Input: part model. Units: mm. Frame: model coordinates. Face numbers are marked on the shaded views. Coordinates: 2 decimals unless noted, no trailing zeros. Write each loop counter-clockwise with the first axis right and the second up, starting at its lowest first coordinate (ties: lowest second). Pieces come first, ordered by that corner, then holes. Notation, with made-up numbers: (72.25, -17.75) - (121.25, -17.75) arc R32 cw to (121.25, 19.25) - close; hole circle Ø4 at (89, 32). An arc over 180 degrees is marked (long way). Put each result on its own line as item: value. Start each with the question number.
1. Cut plane B-B, the plane z = 54.5. Return loops of the section in (x, y).
2. Cut plane C-C, the plane z = -13.5. Return loops of the section in (x, y), and give its area (3 significant figures).
3. Cut plane A-A, the plane y = 0. Return loops of the section in (x, z), and give its area (3 significant figures).
4. Line query: line 1 (Y direction, x = 7.75, z = 0); line 2 (Z direction, x = 14.5, y = -32); line 3 (Z direction, x = 14.25, y = 24.5). Output: solid intervals per line, ascending.
5. Cut plane D-D, the plane x = 11.75. Count the separate pieces of the cut face and the enclosed holes in it, and give its area (3 significant figures).
6. Pull-direction query (Z, two-part tool) for the marked faces 1, 2 and 3; classes: released by +Z, released by -Z, zero draft, split by the parting line, or undercut.
7. Pin query (flat end, axial travel): pin 1 (10 mm diameter, centred on x = 15.5, z = 31, fed in from +Y); pin 2 (3.5 mm diameter, centred on x = 10.5, y = 33.5, fed in from -Z); pin 3 (4 mm diameter, centred on x = 14, z = 30, fed in from +Y). Return the tip coordinate at first contact, or that it passes through.
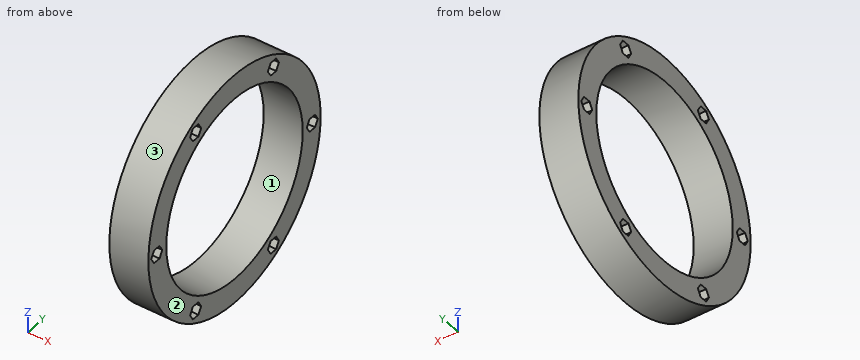
from build123d import *

# Parameters (mm, degrees)
SKETCH1_R           = 72
SKETCH1_R_2         = 57
BOSS_EXTRUDE1_DEPTH = 24
CUT_EXTRUDE1_DEPTH  = 24


with BuildPart() as part:
    # Sketch1 → Boss-Extrude1 (new body)
    with BuildSketch(Plane(origin=(0, 0, 0), x_dir=(0, 0, -1), z_dir=(1, 0, 0))):
        Circle(SKETCH1_R)
        Circle(SKETCH1_R_2, mode=Mode.SUBTRACT)
    extrude(amount=BOSS_EXTRUDE1_DEPTH)

    # Sketch2 → Cut-Extrude1 (cut)
    with BuildSketch(Plane(origin=(24, 0, 0), x_dir=(0, 0, -1), z_dir=(1, 0, 0))):
        Polygon((52.291651246, 30.190598923), (56.291651246, 27.881197846), (60.291651246, 30.190598923), (60.291651246, 34.809401077), (56.291651246, 37.118802154), (52.291651246, 34.809401077), align=None)
        Polygon((0, 60.381197846), (4, 62.690598923), (4, 67.309401077), (0, 69.618802154), (-4, 67.309401077), (-4, 62.690598923), align=None)
        Polygon((52.291651246, -30.190598923), (52.291651246, -34.809401077), (56.291651246, -37.118802154), (60.291651246, -34.809401077), (60.291651246, -30.190598923), (56.291651246, -27.881197846), align=None)
        Polygon((0, -60.381197846), (-4, -62.690598923), (-4, -67.309401077), (0, -69.618802154), (4, -67.309401077), (4, -62.690598923), align=None)
        Polygon((-52.291651246, -30.190598923), (-56.291651246, -27.881197846), (-60.291651246, -30.190598923), (-60.291651246, -34.809401077), (-56.291651246, -37.118802154), (-52.291651246, -34.809401077), align=None)
        Polygon((-52.291651246, 30.190598923), (-52.291651246, 34.809401077), (-56.291651246, 37.118802154), (-60.291651246, 34.809401077), (-60.291651246, 30.190598923), (-56.291651246, 27.881197846), align=None)
    extrude(amount=-CUT_EXTRUDE1_DEPTH, mode=Mode.SUBTRACT)


solid = part.part
Report:
1. outline: (0, -47.05) - (24, -47.05) - (24, -36.08) - (0, -36.08) - close; (0, -28.92) - (24, -28.92) - (24, -16.7) - (0, -16.7) - close; (0, 16.7) - (24, 16.7) - (24, 28.92) - (0, 28.92) - close; (0, 36.08) - (24, 36.08) - (24, 47.05) - (0, 47.05) - close
2. outline: (0, -70.72) - (24, -70.72) - (24, -55.38) - (0, -55.38) - close; (0, 55.38) - (24, 55.38) - (24, 70.72) - (0, 70.72) - close
2. area: 737 mm^2
3. outline: (0, -72) - (24, -72) - (24, -57) - (0, -57) - close; (0, 57) - (24, 57) - (24, 72) - (0, 72) - close
3. area: 720 mm^2
4. line 1: y = -72 to -69.62, -60.38 to -57, 57 to 60.38, 69.62 to 72
4. line 2: z = -64.5 to -60.29, -52.29 to -47.17, 47.17 to 52.29, 60.29 to 64.5
4. line 3: z = -67.7 to -51.47, 51.47 to 67.7
5. separate pieces: 1
5. enclosed holes: 7
5. area: 5,750 mm^2
6. face 1: undercut
6. face 2: zero draft
6. face 3: split by the parting line
7. pin 1: stops at y = 67.14
7. pin 2: stops at z = -64.62
7. pin 3: stops at y = 66.33
